from build123d import *

# Parameters (mm, degrees)
BOSS_EXTRUDE1_DEPTH = 12
FILLET2_R           = 6


with BuildPart() as part:
    # Sketch1 → Boss-Extrude1 (new body)
    with BuildSketch(Plane(origin=(0, -295.781515915, 0), x_dir=(1, 0, 0), z_dir=(0, 1, 0))):
        with BuildLine():
            Line((469.577970857, -27), (469.577970857, -14))
            ThreePointArc((469.577970857, -14), (465.477465793, -4.100505063), (455.577970857, 0))
            Line((455.577970857, 0), (396.577970857, 0))
            ThreePointArc((396.577970857, 0), (386.67847592, -4.100505063), (382.577970857, -14))
            Line((382.577970857, -14), (382.577970857, -27))
            Line((382.577970857, -27), (469.577970857, -27))
        make_face()
    extrude(amount=BOSS_EXTRUDE1_DEPTH)

    # Fillet2
    fillet2_edges = [part.edges().sort_by_distance(p)[0] for p in [
        (465.477465793, -283.781515915, 4.100505063),
        (426.077970857, -283.781515915, 0),
        (386.67847592, -283.781515915, 4.100505063),
        (382.577970857, -283.781515915, 20.5),
        (426.077970857, -283.781515915, 27),
        (469.577970857, -283.781515915, 20.5),
    ]]
    fillet(fillet2_edges, radius=FILLET2_R)


solid = part.part
Geometry: final body of the model. Coordinates: model frame, mm. Give positions to 0.01 mm unless a question says otherwise; leave off trailing zeros. Loops run counter-clockwise (first coordinate to the right, second up) from the corner with the lowest first, then second, coordinate; pieces in that order, holes last. Notation, with made-up numbers: (38.5, -9) - (51.5, -9) arc R28 cw to (51.5, 15) - close; hole circle Ø11 at (20.5, -37). An arc over 180 degrees is marked (long way). One line per question, with ' | ' between items. Start each with the question number.
(1) Ray query, line 1 (Y direction, x = 458.5, z = 2); line 2 (Z direction, x = 390.5, y = -293.5); line 3 (Y direction, x = 413.5, z = 25.75). Return the intervals inside material, ascending. Write a range as from..to.
(2) Section query B-B on y = -289. Return loops of the section in (x, z), then the cut area to 3 significant figures.
(3) Section query A-A on x = 417. Return loops of the section in (y, z).
The answers:
1) line 1: -295.78..-285.65 | line 2: 1.39..27 | line 3: -295.78..-286.12
2) outline: (382.63, 14) arc R13.95 ccw to (396.58, 0.05) - (455.58, 0.05) arc R13.95 ccw to (469.53, 14) - (469.53, 26.95) - (382.63, 26.95) - close | area: 2,250 mm2
3) outline: (-295.78, 0) - (-289.78, 0) arc R6 ccw to (-283.78, 6) - (-283.78, 21) arc R6 ccw to (-289.78, 27) - (-295.78, 27) - close
